Build history of the part. All positions in model axes, mm. Face numbers are marked on the shaded views. Round coordinates to 2 decimals unless told otherwise and drop trailing zeros. Loops run counter-clockwise (first coordinate to the right, second up) from the corner with the lowest first, then second, coordinate; pieces in that order, holes last. Notation, with made-up numbers: (26.25, 50) -> (38.25, 50) arc R26 ccw to (38.25, 72) -> close; hole circle Ø5 at (69.5, 15). An arc over 180 degrees is marked (long way). Put each result on its own line as item: value. Start each with the question number.
```python
from build123d import *


with BuildPart() as part:
    # Esquisse1 → Révolution1 (revolve)
    with BuildSketch(Plane(origin=(0, 0, 0), x_dir=(1, 0, 0), z_dir=(0, 1, 0)), mode=Mode.PRIVATE) as r_volution1_sk:
        with BuildLine():
            Line((2, 40), (-12, 40))
            Line((-12, 40), (-12, 40.1))
            Line((-12, 40.1), (-11.1, 41))
            Line((-11.1, 41), (-3.519615242, 41))
            Line((-3.519615242, 41), (-3, 40.1))
            Line((-3, 40.1), (-0.5, 40.1))
            ThreePointArc((-0.5, 40.1), (-0.146446609, 40.246446609), (0, 40.6))
            Line((0, 40.6), (0, 43))
            Line((0, 43), (2, 45))
            Line((2, 45), (47, 45))
            Line((47, 45), (48, 44))
            Line((48, 44), (48, 43.216633349))
            Line((48, 43.216633349), (2, 40))
        make_face()
    revolve(r_volution1_sk.sketch.rotate(Axis((-32.094260439, 0, 0), (1, 0, 0)), 180), axis=Axis((-32.094260439, 0, 0), (1, 0, 0)))  # turned: the seam where the file's is


solid = part.part
```
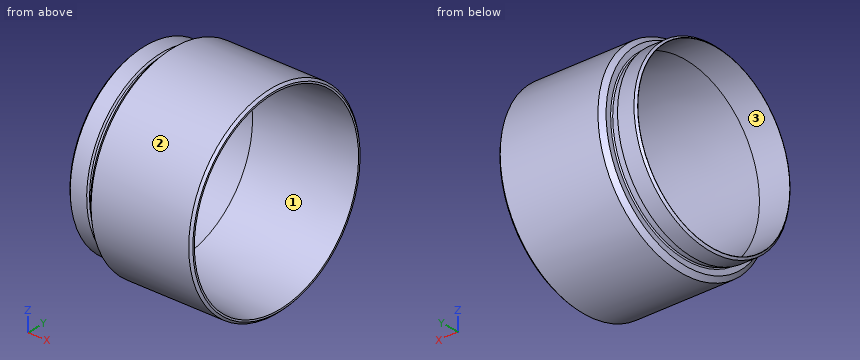
Item 1: Cut at D-D on x = 44. Write the cut outline in (y, z).
Item 2: Drop flat-ended pins along their axis: pin 1 (8 mm diameter, centred on x = 29.5, y = -25, fed in from +Z); pin 2 (3 mm diameter, centred on x = 1.5, z = -8, fed in from -Y); pin 3 (6 mm diameter, centred on x = 33.5, y = 21.5, fed in from -Z). Give the stop position or say it passes through.
Item 3: Cut at C-C on x = 28.5. Write the cut outline in (y, z), then the cut area to 3 significant figures.
Item 4: Wall check: line 1 (Y direction, x = -4, z = 0); line 2 (Y direction, x = 23.5, z = -27.5); line 3 (Z direction, x = 11, y = 13). Give the ranges that are in metal, low to high. Write a range as from..to.
Item 5: Pull direction Z, two halves, no side cores. Call the marked faces 1, 2 and 3: +Z half, -Z half, draft (parallel to the pull), parting line (faces both ways), or undercut.
Item 6: Cut at B-B on z = 0. Write the cut outline in (x, y), then the cut area to 3 significant figures.
Ans:
1. outline: circle Ø90 at (0, 0); hole circle Ø85.87 at (0, 0)
2. pin 1: stops at z = 39.8
2. pin 2: stops at y = -44.52
2. pin 3: stops at z = -41.02
3. outline: circle Ø90 at (0, 0); hole circle Ø83.71 at (0, 0)
3. area: 859 mm2
4. line 1: y = -41..-40, 40..41
4. line 2: y = -35.62..-31.09, 31.09..35.62
4. line 3: z = -43.08..-38.49, 38.49..43.08
5. face 1: undercut
5. face 2: parting line
5. face 3: undercut
6. outline: (-12, -40.1) -> (-11.1, -41) -> (-3.52, -41) -> (-3, -40.1) -> (-0.5, -40.1) arc R0.5 cw to (0, -40.6) -> (0, -43) -> (2, -45) -> (47, -45) -> (48, -44) -> (48, -43.22) -> (2, -40) -> (-12, -40) -> close; (-12, 40) -> (2, 40) -> (48, 43.22) -> (48, 44) -> (47, 45) -> (2, 45) -> (0, 43) -> (0, 40.6) arc R0.5 cw to (-0.5, 40.1) -> (-3, 40.1) -> (-3.52, 41) -> (-11.1, 41) -> (-12, 40.1) -> close
6. area: 344 mm2
